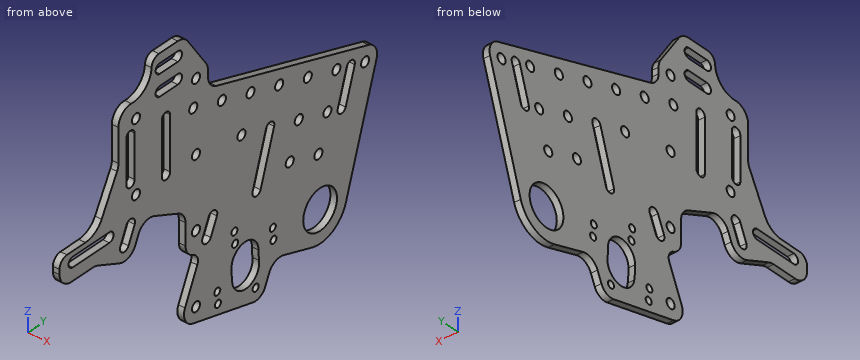
```python
from build123d import *

# Parameters (mm, degrees)
SKETCH2_R           = 14.2875
SKETCH2_R_2         = 3.429
SKETCH2_R_3         = 2.54
BOSS_EXTRUDE1_DEPTH = 4.7625


with BuildPart() as part:
    # Sketch2 → Boss-Extrude1 (new body)
    with BuildSketch(Plane(origin=(0, 0, 0), x_dir=(0, 0, -1), z_dir=(1, 0, 0))):
        with BuildLine():
            Line((38.021448917, 246.234864084), (120.241230069, 220.311066665))
            ThreePointArc((120.241230069, 220.311066665), (133.644163138, 209.06467047), (135.169064986, 191.634962595))
            Line((135.169064986, 191.634962595), (127.622152065, 167.6992128))
            ThreePointArc((127.622152065, 167.6992128), (128.044603019, 160.47960856), (133.162508812, 155.36999111))
            Line((133.162508812, 155.36999111), (140.48887895, 152.092017357))
            ThreePointArc((140.48887895, 152.092017357), (144.852236282, 147.866521475), (145.483799346, 141.825426314))
            Line((145.483799346, 141.825426314), (132.821367632, 91.06703794))
            ThreePointArc((132.821367632, 91.06703794), (127.408392323, 84.390132513), (118.814072234, 84.252183312))
            Line((118.814072234, 84.252183312), (95.644233558, 94.61886171))
            ThreePointArc((95.644233558, 94.61886171), (90.786060122, 94.754966448), (87.254572158, 91.415959651))
            Line((87.254572158, 91.415959651), (86.910445683, 90.646826606))
            ThreePointArc((86.910445683, 90.646826606), (83.162135594, 86.27028604), (77.636394916, 84.636234079))
            Line((77.636394916, 84.636234079), (62.21871433, 84.636234079))
            ThreePointArc((62.21871433, 84.636234079), (56.692973652, 83.002182118), (52.944663563, 78.625641552))
            Line((52.944663563, 78.625641552), (43.839685496, 58.275741142))
            ThreePointArc((43.839685496, 58.275741142), (43.621917914, 50.502663645), (48.96432879, 44.852282903))
            Line((48.96432879, 44.852282903), (54.760610519, 42.258903232))
            ThreePointArc((54.760610519, 42.258903232), (60.103021394, 36.60852249), (59.885253813, 28.835444993))
            Line((59.885253813, 28.835444993), (51.685949233, 10.509752126))
            ThreePointArc((51.685949233, 10.509752126), (51.023955621, 8.481811623), (50.8, 6.360344653))
            Line((50.8, 6.360344653), (50.8, -11.7475))
            ThreePointArc((50.8, -11.7475), (47.824204897, -18.931704897), (40.64, -21.9075))
            Line((40.64, -21.9075), (37.1475, -21.9075))
            ThreePointArc((37.1475, -21.9075), (32.657371939, -20.047628061), (30.7975, -15.5575))
            Line((30.7975, -15.5575), (30.7975, 0))
            ThreePointArc((30.7975, 0), (28.552596998, 8.032774411), (22.468409419, 13.737834946))
            Line((22.468409419, 13.737834946), (-2.554479623, 26.788416358))
            ThreePointArc((-2.554479623, 26.788416358), (-4.834094275, 27.647905305), (-7.252780881, 27.94))
            Line((-7.252780881, 27.94), (-31.256978796, 27.94))
            ThreePointArc((-31.256978796, 27.94), (-38.707276299, 31.19213006), (-41.38801938, 38.866561592))
            ThreePointArc((-41.38801938, 38.866561592), (-45.28789684, 50.537792221), (-56.355984579, 55.915905494))
            ThreePointArc((-56.355984579, 55.915905494), (-60.621662669, 57.889989399), (-62.361270294, 62.25654206))
            Line((-62.361270294, 62.25654206), (-62.361270294, 78.164314079))
            ThreePointArc((-62.361270294, 78.164314079), (-61.17251471, 82.933210558), (-57.884425091, 86.586151856))
            Line((-57.884425091, 86.586151856), (-35.119675091, 101.948071856))
            ThreePointArc((-35.119675091, 101.948071856), (-32.408029017, 103.24198088), (-29.436520294, 103.686234079))
            Line((-29.436520294, 103.686234079), (-25.026637608, 103.686234079))
            ThreePointArc((-25.026637608, 103.686234079), (-19.01893158, 105.6527569), (-15.336873388, 110.791063156))
            Line((-15.336873388, 110.791063156), (25.276513775, 239.600270788))
            ThreePointArc((25.276513775, 239.600270788), (30.274912084, 245.55712993), (38.021448917, 246.234864084))
        make_face()
        with Locations((113.367095492, 198.509097171)):
            Circle(SKETCH2_R, mode=Mode.SUBTRACT)
        with Locations((-29.436520294, 42.726234079)):
            Circle(SKETCH2_R_2, mode=Mode.SUBTRACT)
        with Locations((21.363479706, 93.526234079)):
            Circle(SKETCH2_R_2, mode=Mode.SUBTRACT)
        with Locations((122.963479706, 93.526234079)):
            Circle(SKETCH2_R_2, mode=Mode.SUBTRACT)
        with Locations((104.398969727, 158.50014909)):
            Circle(SKETCH2_R_3, mode=Mode.SUBTRACT)
        with Locations((136.858147411, 143.977222936)):
            Circle(SKETCH2_R_3, mode=Mode.SUBTRACT)
        with Locations((122.335221257, 111.518045252)):
            Circle(SKETCH2_R_3, mode=Mode.SUBTRACT)
        with Locations((89.876043573, 126.040971407)):
            Circle(SKETCH2_R_3, mode=Mode.SUBTRACT)
        with Locations((112.840572264, 159.063757816)):
            Circle(SKETCH2_R_3, mode=Mode.SUBTRACT)
        with Locations((130.776823793, 112.081653978)):
            Circle(SKETCH2_R_3, mode=Mode.SUBTRACT)
        with Locations((98.317646109, 126.604580132)):
            Circle(SKETCH2_R_3, mode=Mode.SUBTRACT)
        with Locations((-29.436520294, 93.526234079)):
            Circle(SKETCH2_R_2, mode=Mode.SUBTRACT)
        with Locations((21.363479706, 42.726234079)):
            Circle(SKETCH2_R_2, mode=Mode.SUBTRACT)
        with Locations((72.163479706, 93.526234079)):
            Circle(SKETCH2_R_2, mode=Mode.SUBTRACT)
        with Locations((34.966277994, 236.545099865)):
            Circle(SKETCH2_R_2, mode=Mode.SUBTRACT)
        with Locations((27.328350687, 212.320689316)):
            Circle(SKETCH2_R_2, mode=Mode.SUBTRACT)
        with Locations((19.690423379, 188.096278767)):
            Circle(SKETCH2_R_2, mode=Mode.SUBTRACT)
        with Locations((12.052496072, 163.871868218)):
            Circle(SKETCH2_R_2, mode=Mode.SUBTRACT)
        with Locations((4.414568765, 139.647457669)):
            Circle(SKETCH2_R_2, mode=Mode.SUBTRACT)
        with Locations((-3.223358543, 115.42304712)):
            Circle(SKETCH2_R_2, mode=Mode.SUBTRACT)
        with Locations((-10.86128585, 91.198636571)):
            Circle(SKETCH2_R_2, mode=Mode.SUBTRACT)
        with Locations((51.552761236, 204.682762008)):
            Circle(SKETCH2_R_2, mode=Mode.SUBTRACT)
        with Locations((43.914833928, 180.458351459)):
            Circle(SKETCH2_R_2, mode=Mode.SUBTRACT)
        with Locations((75.777171785, 197.044834701)):
            Circle(SKETCH2_R_2, mode=Mode.SUBTRACT)
        with Locations((68.139244477, 172.820424152)):
            Circle(SKETCH2_R_2, mode=Mode.SUBTRACT)
        with Locations((28.638979314, 132.009530361)):
            Circle(SKETCH2_R_2, mode=Mode.SUBTRACT)
        with BuildLine():
            Line((30.078004517, 221.041477113), (54.302415066, 213.403549806))
            ThreePointArc((54.302415066, 213.403549806), (58.763142366, 215.72565746), (56.441034713, 220.18638476))
            Line((56.441034713, 220.18638476), (32.216624164, 227.824312067))
            ThreePointArc((32.216624164, 227.824312067), (27.755896864, 225.502204413), (30.078004517, 221.041477113))
        make_face(mode=Mode.SUBTRACT)
        with BuildLine():
            Line((41.656, 20.2565), (41.656, -10.7315))
            ThreePointArc((41.656, -10.7315), (38.1, -14.2875), (34.544, -10.7315))
            Line((34.544, -10.7315), (34.544, 20.2565))
            ThreePointArc((34.544, 20.2565), (38.1, 23.8125), (41.656, 20.2565))
        make_face(mode=Mode.SUBTRACT)
        with BuildLine():
            Line((-20.2565, 41.656), (10.7315, 41.656))
            ThreePointArc((10.7315, 41.656), (14.2875, 38.1), (10.7315, 34.544))
            Line((10.7315, 34.544), (-20.2565, 34.544))
            ThreePointArc((-20.2565, 34.544), (-23.8125, 38.1), (-20.2565, 41.656))
        make_face(mode=Mode.SUBTRACT)
        with BuildLine():
            Line((-48.645270294, 78.164314079), (-48.645270294, 62.924314079))
            ThreePointArc((-48.645270294, 62.924314079), (-52.201270294, 59.368314079), (-55.757270294, 62.924314079))
            Line((-55.757270294, 62.924314079), (-55.757270294, 78.164314079))
            ThreePointArc((-55.757270294, 78.164314079), (-52.201270294, 81.720314079), (-48.645270294, 78.164314079))
        make_face(mode=Mode.SUBTRACT)
        with BuildLine():
            Line((-33.405270294, 78.164314079), (-33.405270294, 62.924314079))
            ThreePointArc((-33.405270294, 62.924314079), (-36.961270294, 59.368314079), (-40.517270294, 62.924314079))
            Line((-40.517270294, 62.924314079), (-40.517270294, 78.164314079))
            ThreePointArc((-40.517270294, 78.164314079), (-36.961270294, 81.720314079), (-33.405270294, 78.164314079))
        make_face(mode=Mode.SUBTRACT)
        with BuildLine():
            Line((37.346216444, 159.625358387), (73.682832268, 148.168467426))
            ThreePointArc((73.682832268, 148.168467426), (76.004939921, 143.707740126), (71.544212621, 141.385632472))
            Line((71.544212621, 141.385632472), (35.207596798, 152.842523433))
            ThreePointArc((35.207596798, 152.842523433), (32.885489144, 157.303250733), (37.346216444, 159.625358387))
        make_face(mode=Mode.SUBTRACT)
        with BuildLine():
            Line((-16.736520294, 71.682234079), (21.363479706, 71.682234079))
            ThreePointArc((21.363479706, 71.682234079), (24.919479706, 68.126234079), (21.363479706, 64.570234079))
            Line((21.363479706, 64.570234079), (-16.736520294, 64.570234079))
            ThreePointArc((-16.736520294, 64.570234079), (-20.292520294, 68.126234079), (-16.736520294, 71.682234079))
        make_face(mode=Mode.SUBTRACT)
        with BuildLine():
            Line((71.695223435, 111.204761595), (83.287786894, 106.018002254))
            ThreePointArc((83.287786894, 106.018002254), (85.209528129, 100.984205414), (80.175731289, 99.062464179))
            Line((80.175731289, 99.062464179), (68.583167831, 104.24922352))
            ThreePointArc((68.583167831, 104.24922352), (66.661426596, 109.28302036), (71.695223435, 111.204761595))
        make_face(mode=Mode.SUBTRACT)
        with BuildLine():
            Line((40.57466739, 41.649380844), (52.167230848, 36.462621503))
            ThreePointArc((52.167230848, 36.462621503), (54.088972084, 31.428824663), (49.055175244, 29.507083428))
            Line((49.055175244, 29.507083428), (37.462611785, 34.693842769))
            ThreePointArc((37.462611785, 34.693842769), (35.54087055, 39.727639609), (40.57466739, 41.649380844))
        make_face(mode=Mode.SUBTRACT)
        with BuildLine():
            ThreePointArc((112.879749334, 123.580682042), (118.115569936, 123.729709032), (123.328186485, 124.244155468))
            ThreePointArc((123.328186485, 124.244155468), (133.137248458, 137.092194354), (120.289209572, 146.901256326))
            ThreePointArc((120.289209572, 146.901256326), (116.666882818, 146.543759651), (113.028431213, 146.440198522))
            ThreePointArc((113.028431213, 146.440198522), (101.524332034, 135.084781222), (112.879749334, 123.580682042))
        make_face(mode=Mode.SUBTRACT)
    extrude(amount=BOSS_EXTRUDE1_DEPTH)


solid = part.part
```
CAD build for the part. Positions are in the model's coordinates, mm. Round coordinates to 2 decimals unless told otherwise and drop trailing zeros.
Q1. Slice it at A-A (x = 3.35). State how many separate pieces and enclosed holes the cut face has, and give its area (3 significant figures).
Q2. Wall check: L1, parallel to Z at x = 1.65, y = 127.5; L2, parallel to Y at x = 1.25, z = -105.5; L3, parallel to Y at x = 4.3, z = -116. Give the ranges that are in metal, low to high.
Q3. Drop flat-ended pins along their axis: pin 1 (1.4 mm diameter, centred on x = 2, y = -11.5, fed in from +Z); pin 2 (1.5 mm diameter, centred on x = 1, y = 203.5, fed in from +Z); pin 3 (1.4 mm diameter, centred on x = 1.5, z = 6, fed in from -Y). Give the stop position or say it passes through.
Results below:
1. separate pieces: 1
1. enclosed holes: 36
1. area: 23,700 mm2
2. L1: z = -141.91 to -129.9, -104.34 to -100.69, -95.94 to -91.96, -87.8 to 10.07
2. L2: y = 90.21 to 126.35, 143.68 to 156.21, 160.79 to 186.58, 210.44 to 224.96
2. L3: y = 85.51 to 123.63, 146.51 to 184.47, 212.55 to 221.65
3. pin 1: stops at z = -30.8
3. pin 2: stops at z = -13.66
3. pin 3: stops at y = 27.75
